The drawing under review shows one solid part. Ordinate dimensions are in mm from its lowest x, y, z. A direction names the side the tool comes from. Coordinates: 2 decimals unless noted, no trailing zeros. Write each loop counter-clockwise with the first axis right and the second up, starting at its lowest first coordinate (ties: lowest second). Pieces come first, ordered by that corner, then holes. Notation, with made-up numbers: M -36,-6.75 L -21,-6.75 A15 cw -21,18.25 Z; hole C 25.5,45.5 d3. An arc over 180 degrees is marked long. Write item = value, one per line.
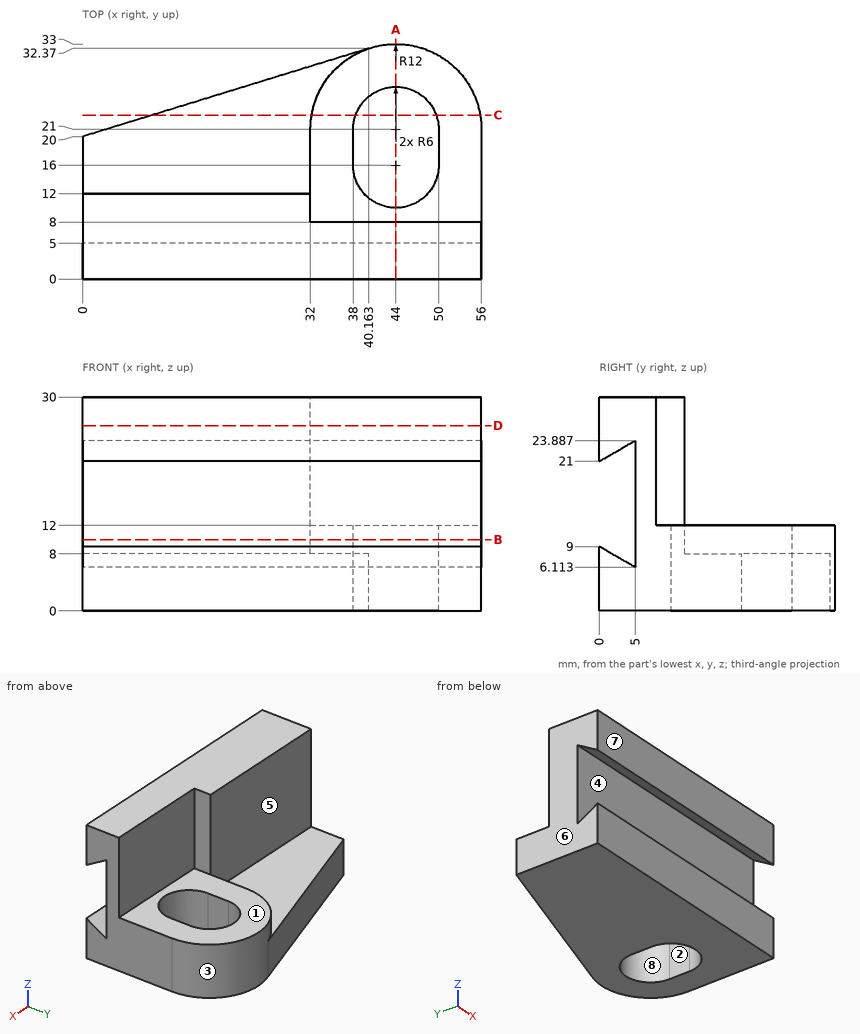
Q1. Consider section A-A, the plane x = 44. State the section outline as (y, z) points.
Check result:
outline = M 0,0 L 10,0 L 10,12 L 8,12 L 8,30 L 0,30 L 0,21 L 5,23.89 L 5,6.11 L 0,9 Z; M 27,0 L 33,0 L 33,12 L 27,12 Z
Q2. Consider section D-D, the plane z = 26. State the section outline as (x, y) points.
Check result:
outline = M 0,0 L 56,0 L 56,8 L 32,8 L 32,12 L 0,12 Z
Q3. Consider section C-C, the plane y = 23. State the section outline as (x, z) points.
Check result:
outline = M 9.74,0 L 38.34,0 L 38.34,12 L 32.17,12 L 32.17,8 L 9.74,8 Z; M 49.66,0 L 55.83,0 L 55.83,12 L 49.66,12 Z
Q4. The part is to be moulded in two halves that separate along Y. For the marked faces 6, 7 and 8, say which applies: +Y half, -Y half, draft (parallel to the pull), parting line (faces both ways), or undercut.
Check result:
face_6 = draft
face_7 = -Y half
face_8 = undercut
Q5. Consider section B-B, the plane z = 10. State the section outline as (x, y) points, and give its area (3 significant figures).
Check result:
outline = M 0,5 L 56,5 L 56,21 A12 ccw 32,21 L 32,12 L 0,12 Z; hole M 38,16 A6 ccw 50,16 L 50,21 A6 ccw 38,21 Z
area = 661 mm²
Q6. Machinability: for the marked faces 1, 2, 3, 4 and 5, which of the approach directions +Z, -Z, +X, -X, +Y, -Y give a long, thin tool a straight path to every point of the face, cutting with its end or side? Answer none if there is none.
Check result:
face_1 = +Z, +X, +Y
face_2 = +Z, -Z
face_3 = +Z, +Y
face_4 = +X, -X
face_5 = +Z, -X, +Y
Q7. For P1, Ø9, axis at x = 42, z = 14.5, coming from the -Y side; P2, Ø4, axis at x = 11, z = 14.5, coming from the +Y side; P3, Ø10, axis at x = 24.5, y = 19, coming from the +Z side, all flat-tipped, find the tip position at first contact; note any pin that passes through.
Check result:
P1 = 5
P2 = 12
P3 = 8
Q8. Wall thickness on line 1 (X direction, y = 17, z = 10.5); line 2 (X direction, y = 10.5, z = 23); line 3 (Y direction, x = 30.5, z = 19.25): over which ranges is each line inside the solid? List them lowest first.
Check result:
line_1 = 32 to 38, 50 to 56
line_2 = 0 to 32
line_3 = 5 to 12
